The model under review builds one solid part; all positions refer to its coordinate system, in mm. A direction names the side the tool comes from. Give positions to 0.01 mm unless a question says otherwise; leave off trailing zeros. Loops run counter-clockwise (first coordinate to the right, second up) from the corner with the lowest first, then second, coordinate; pieces in that order, holes last. Notation, with made-up numbers: (-40, 89) - (-18, 89) arc R14 ccw to (-18, 106) - close; hole circle Ø3 at (6, 64.5). An arc over 180 degrees is marked (long way). Answer as a JSON object with one key per item and string values.
from build123d import *

# Parameters (mm, degrees)
SKETCH_1_W          = 40
SKETCH_1_H          = 20
SKETCH_1_W_2        = 36
SKETCH_1_H_2        = 16
EXTRUDE_1_DEPTH     = 50
SKETCH_2_R          = 1.45
CUT_EXTRUDE_1_DEPTH = 65.807406984
SKETCH_3_R          = 1.5
CUT_EXTRUDE_2_DEPTH = 58.445626465
SKETCH_4_R          = 1.5
CUT_EXTRUDE_3_DEPTH = 58.445626465


with BuildPart() as part:
    # 草图1 → 凸台-拉伸1 (new, symmetric)
    with BuildSketch(Plane(origin=(0, 0, 0), x_dir=(1, 0, 0), z_dir=(0, 1, 0))):
        Rectangle(SKETCH_1_W, SKETCH_1_H)
        Rectangle(SKETCH_1_W_2, SKETCH_1_H_2, mode=Mode.SUBTRACT)
    extrude(amount=EXTRUDE_1_DEPTH, both=True)

    # 草图2 → 切除-拉伸1 (cut, through all)
    with BuildSketch(Plane(origin=(20, 0, 0), x_dir=(0, 0, -1), z_dir=(1, 0, 0))):
        with Locations((5, 45)):
            Circle(SKETCH_2_R)
        with Locations((-5, 45)):
            Circle(SKETCH_2_R)
        with Locations((5, 0)):
            Circle(SKETCH_2_R)
        with Locations((-5, 0)):
            Circle(SKETCH_2_R)
        with Locations((5, -45)):
            Circle(SKETCH_2_R)
        with Locations((-5, -45)):
            Circle(SKETCH_2_R)
    extrude(amount=-CUT_EXTRUDE_1_DEPTH, mode=Mode.SUBTRACT)

    # 草图3 → 切除-拉伸2 (cut, through all)
    with BuildSketch(Plane(origin=(0, 0, -10), x_dir=(-1, 0, 0), z_dir=(0, 0, -1))):
        with Locations((10, 35)):
            Circle(SKETCH_3_R)
        with Locations((0, 35)):
            Circle(SKETCH_3_R)
        with Locations((-10, 35)):
            Circle(SKETCH_3_R)
    extrude(amount=-CUT_EXTRUDE_2_DEPTH, mode=Mode.SUBTRACT)

    # 草图4 → 切除-拉伸3 (cut, through all)
    with BuildSketch(Plane(origin=(0, 0, -10), x_dir=(-1, 0, 0), z_dir=(0, 0, -1))):
        with Locations((0, -45)):
            Circle(SKETCH_4_R)
        with Locations((-10, -45)):
            Circle(SKETCH_4_R)
        with Locations((9.9, -22.0875)):
            Circle(SKETCH_4_R)
    extrude(amount=-CUT_EXTRUDE_3_DEPTH, mode=Mode.SUBTRACT)


solid = part.part
Q1. Consider section B-B, the plane x = -15. State the section outline as (y, z) points, plus the area to 3 significant figures.
Results:
{"outline": "(-50, -10) - (50, -10) - (50, -8) - (-50, -8) - close; (-50, 8) - (50, 8) - (50, 10) - (-50, 10) - close", "area": "400 mm^2"}
Q2. Consider section D-D, the plane y = 45. State the section outline as (x, z) points.
Results:
{"outline": "(-20, -10) - (20, -10) - (20, -6.45) - (18, -6.45) - (18, -8) - (-18, -8) - (-18, -6.45) - (-20, -6.45) - close; (-20, -3.55) - (-18, -3.55) - (-18, 3.55) - (-20, 3.55) - close; (-20, 6.45) - (-18, 6.45) - (-18, 8) - (18, 8) - (18, 6.45) - (20, 6.45) - (20, 10) - (-20, 10) - close; (18, -3.55) - (20, -3.55) - (20, 3.55) - (18, 3.55) - close"}
Q3. To check wall thickness, follow probe 1 along Y at (x, z) = (-18.9, -5); probe 2 along Y at (x, z) = (10, -9.3); probe 3 along Z at (x, y) = (2, 22). State the ranges of each line that lie inside material, in increasing order. Write a range as [from, to].
Results:
{"probe 1": "y = [-50, -46.45], [-43.55, -1.45], [1.45, 43.55], [46.45, 50]", "probe 2": "y = [-50, -46.5], [-43.5, 33.5], [36.5, 50]", "probe 3": "z = [-10, -8], [8, 10]"}
Q4. Consider section C-C, the plane z = 5. State how many separate pieces and enclosed holes the cut face has, plus the area to 3 significant figures.
Results:
{"separate pieces": "8", "enclosed holes": "0", "area": "365 mm^2"}
Q5. The part is to be moulded in two halves that separate along Y. For faces 1 (the face through (0, 1, 10)), 2 (the face through (19.01, 0.06, 6.45)), 3 (the face through (-18.99, 0.06, 6.45)), 4 (the face through (-0.1, 50, -8.2)), say which applies: +Y half, -Y half, draft (parallel to the pull), parting line (faces both ways), or undercut.
Results:
{"face 1": "draft", "face 2": "undercut", "face 3": "undercut", "face 4": "+Y half"}
Q6. For faces 5 (the face through (0, 1, 8)), 6 (the face through (-18.99, 0.06, -3.55)), list the 3-axis set-ups (+Z, -Z, +X, -X, +Y, -Y) from which the entire face can be reached by the end or side of a thin tool; tool diameter is ignored.
Results:
{"face 5": "+Y, -Y", "face 6": "+X, -X"}
Q7. Consider section A-A, the plane z = -2. State the section outline as (x, y) points.
Results:
{"outline": "(-20, -50) - (-18, -50) - (-18, 50) - (-20, 50) - close; (18, -50) - (20, -50) - (20, 50) - (18, 50) - close"}
